Design review of the part shown in the three views and the two pictorial views. Dimensions are in mm from the part's minimum x, y and z. Give positions to 0.01 mm unless a question says otherwise; leave off trailing zeros. Order: outer loops, then holes, each group sorted by start corner. A loop starts at its lowest first (then second) coordinate and runs counter-clockwise, first axis right, second up. Notation, with made-up numbers: (4.25, -36.75) - (55.25, -36.75) arc R15 ccw to (55.25, -8.75) - close; hole circle Ø3 at (58, 55.25). An arc over 180 degrees is marked (long way). Put each result on its own line as item: value. Start each with the question number.
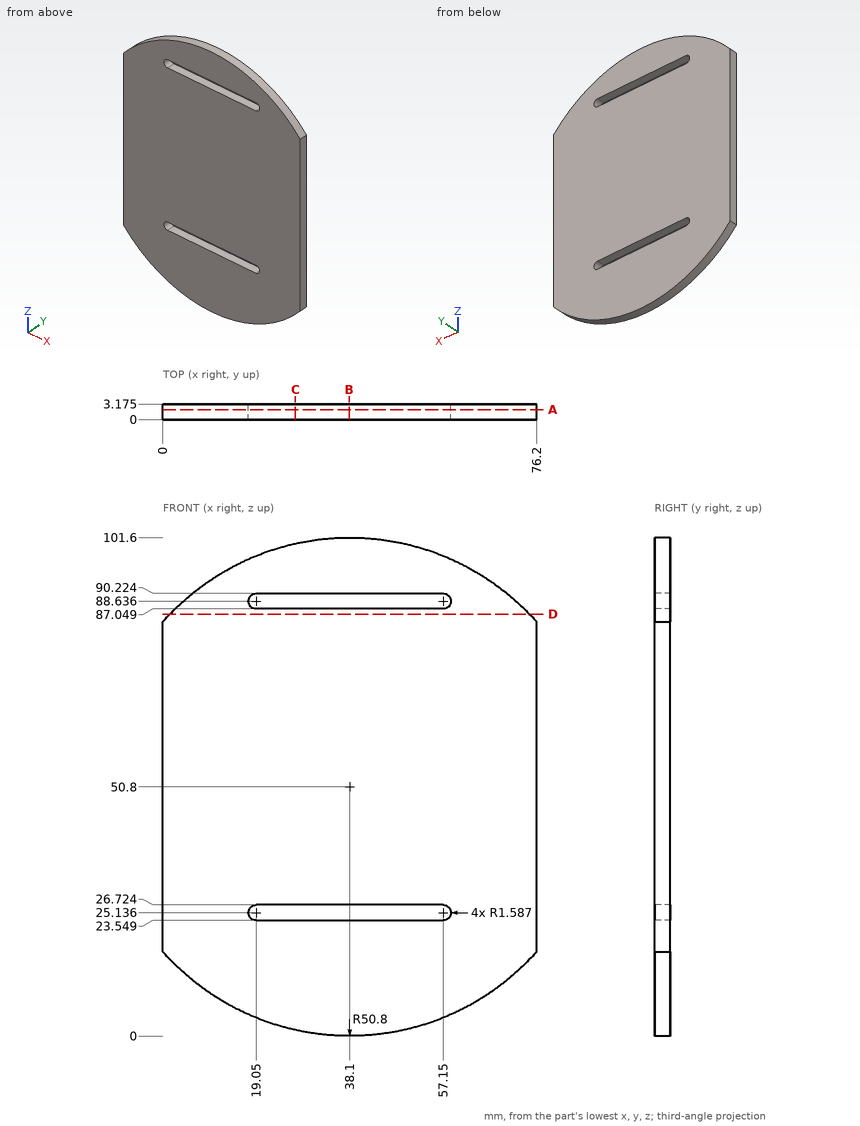
1. Add section D-D, the plane z = 86. Give the boundary of the cut face in (x, y) (1 decimal).
2. Add section A-A, the plane y = 2.05. Count the separate pieces of the cut face and the enclosed holes in it, then the cut area to 3 significant figures.
3. Clearance check with flat-ended pins moving along their axes: pin 1 (1.6 mm diameter, centred on x = 35.5, y = 2, fed in from -Z); pin 2 (1 mm diameter, centred on x = 33, y = 2, fed in from -Z); pin 3 (1.5 mm diameter, centred on y = 2, z = 85.5, fed in from +X). State where each tip first meets the part, or that it passes through.
4. Add section B-B, the plane x = 38. Give the boundary of the cut face in (y, z) (1 decimal).
5. Wall thickness on line 1 (X direction, y = 0.8, z = 92) (1 decimal); line 2 (Z direction, x = 67, y = 1.4); line 3 (X direction, y = 2.1, z = 95): over which ranges is each line inside the solid? List them lowest first. Write a range as from..to.
6. Add section C-C, the plane x = 27. Give the boundary of the cut face in (y, z) (1 decimal).
Found:
1. outline: (1.5, 0) - (74.7, 0) - (74.7, 3.2) - (1.5, 3.2) - close
2. separate pieces: 1
2. enclosed holes: 2
2. area: 6,680 mm^2
3. pin 1: stops at z = 0.03
3. pin 2: stops at z = 0.21
3. pin 3: stops at x = 75.89
4. outline: (0, 0) - (3.2, 0) - (3.2, 23.5) - (0, 23.5) - close; (0, 26.7) - (3.2, 26.7) - (3.2, 87) - (0, 87) - close; (0, 90.2) - (3.2, 90.2) - (3.2, 101.6) - (0, 101.6) - close
5. line 1: x = 8.4..67.8
5. line 2: z = 9.02..92.58
5. line 3: x = 13.06..63.14
6. outline: (0, 1.2) - (3.2, 1.2) - (3.2, 23.5) - (0, 23.5) - close; (0, 26.7) - (3.2, 26.7) - (3.2, 87) - (0, 87) - close; (0, 90.2) - (3.2, 90.2) - (3.2, 100.4) - (0, 100.4) - close
